Check sheet for the modelled part. Datum: model origin and axes. Units: mm. Face numbers are marked on the shaded views. A direction names the side the tool comes from. Give positions to 0.01 mm unless a question says otherwise; leave off trailing zeros. Order: outer loops, then holes, each group sorted by start corner. A loop starts at its lowest first (then second) coordinate and runs counter-clockwise, first axis right, second up. Notation, with made-up numbers: (6.5, 48) -> (58.5, 48) arc R20 cw to (58.5, 61) -> close; hole circle Ø8 at (69, 64.25). An arc over 180 degrees is marked (long way). One line per question, with ' | ' between items.
```python
from build123d import *

# Parameters (mm, degrees)
F2_R    = 10.614455
F3_SIZE = 5


with BuildPart() as f1:
    # F0 (on Front) → F1 (revolve)
    with BuildSketch(Plane.XZ):
        Polygon((-98.246373, 0), (0, 0), (0, 76.596335), (-31.355228, 76.596335), (-31.355228, 47.630079), (-40.911108, 47.630079), (-40.911108, 61.068039), (-54.647684, 61.068039), (-81.52359, 42.852145), (-81.52359, 20.156933), (-90.183608, 20.156933), (-90.183608, 39.268687), (-98.246373, 39.268687), align=None)
    revolve(axis=Axis((-49.123187, 0, 0), (-1, 0, 0)))

    # F2
    f2_edges = [f1.edges().sort_by_distance(p)[0] for p in [
        (-81.52359, 0, -42.852145),
    ]]
    fillet(f2_edges, radius=F2_R)

    # F3
    f3_edges = [f1.edges().sort_by_distance(p)[0] for p in [
        (-31.355228, 0, -76.596335),
    ]]
    chamfer(f3_edges, length=F3_SIZE)

    # F4: F1 across face


with BuildPart() as f1_1:
    add(f1.part)
    add(f1.part.mirror(Plane.YZ))

    # F5: F1 across plane


with BuildPart() as f1_2:
    add(f1_1.part)
    add(f1_1.part.mirror(Plane.YZ))


solid = f1_2.part
```
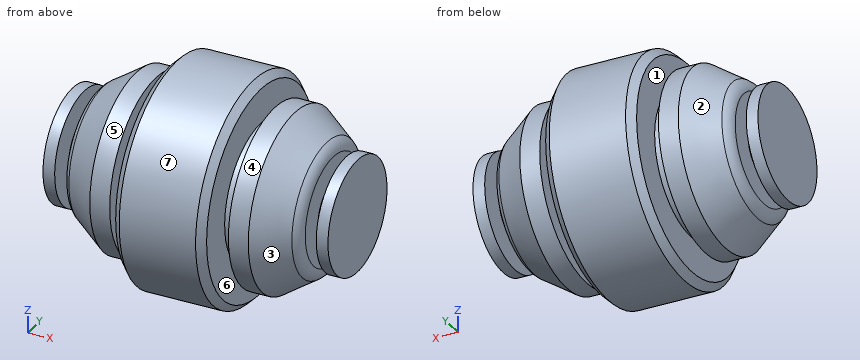
Q1. Section check C-C (x = 63). Enter the section's corners in (y, z).
Result sheet:
outline: circle Ø110.81 at (0, 0)
Q2. Section check A-A (z = 52). Count the separate pieces of the cut face and the enclosed holes in it, and give its area (3 significant figures).
Result sheet:
separate pieces: 3 | enclosed holes: 0 | area: 9,870 mm2
Q3. Thickness scan on line 1 (X direction, y = -15, z = 23); line 2 (X direction, y = 52.5, z = 29); line 3 (X direction, y = -35, z = -50.5). Record the ranges inside material, lowest first.
Result sheet:
line 1: x = -98.25 to -90.18, -81.52 to 81.52, 90.18 to 98.25 | line 2: x = -56.26 to -40.91, -31.36 to 31.36, 40.91 to 56.26 | line 3: x = -31.36 to 31.36
Q4. Access from +Z, -Z, +X, -X, +Y, -Y to the whole of each face (thin tool, end or side, straight path). Record for the marked faces 5, 6 and 7.
Result sheet:
face 5: -X | face 6: none | face 7: +X, -X
Q5. Mould release check, pull along X, two halves, no side actions. Record for the marked faces 1, 2, 3 and 4: pulls with the +X half, pulls with the -X half, needs draft (parallel to the pull), parting line crosses it, or undercut.
Result sheet:
face 1: undercut | face 2: pulls with the -X half | face 3: pulls with the +X half | face 4: needs draft
Q6. Depth check by flat-ended pin: pin 1 Ø2 at (x, z) = (-42.5, 42.5) entering from +Y; pin 2 Ø4 at (y, z) = (35.5, 21.5) entering from -X; pin 3 Ø2 at (x, z) = (76.5, 14.5) entering from +Y. Enter the tip coordinate at first touch or a pass-through.
Result sheet:
pin 1: stops at y = 44.8 | pin 2: stops at x = -81.28 | pin 3: stops at y = 44.71
